Can you work these out from the model? Positions are in its coordinate system, mm. Face numbers are marked on the shaded views. Give positions to 0.01 mm unless a question says otherwise; leave off trailing zeros. Order: outer loops, then holes, each group sorted by start corner. A loop starts at its lowest first (then second) coordinate and runs counter-clockwise, first axis right, second up. Notation, with made-up numbers: (32, -27) - (61, -27) arc R18 ccw to (61, 8) - close; hole circle Ø3 at (-7.75, 84.25). An arc over 180 degrees is marked (long way). Use one line per item in the form item = value. Start each with the question number.
1) We'd pull the mould along X, two halves only. Please class the marked faces 1 and 2: released by +X, released by -X, zero draft, split by the parting line, or undercut.
2) For pin 1 (5 mm diameter, centred on x = 200, z = -85, fed in from +Y); pin 2 (9 mm diameter, centred on x = 404.2, z = -85, fed in from -Y), each with a flat end and sliding along its axis, tell me the tip position at first contact or that it passes through.
3) Suppose I cut it at A-A, the plane z = -65. Write out the boundary of the cut face in (x, y).
4) Suppose I cut it at B-B, the plane x = 52.5. Write out the boundary of the cut face in (y, z), and give its area (3 significant figures).
5) Please list where these lines run through material, in increasing order: probe 1 along X at (y, z) = (5.75, -15); probe 2 along X at (y, z) = (-1.75, -74.5); probe 3 along Z at (x, y) = (200, 6).
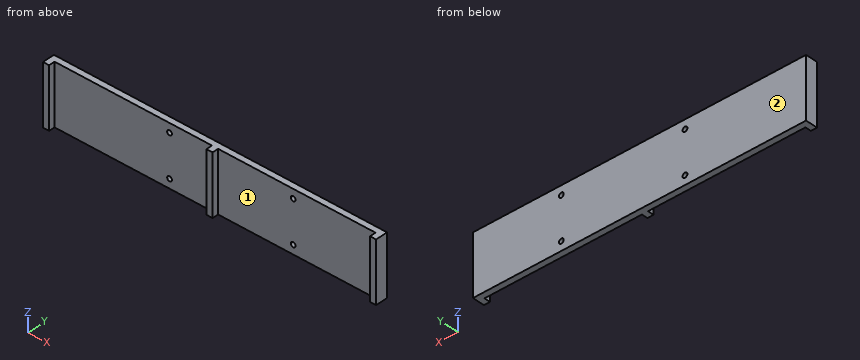
```python
from build123d import *

# Parameters (mm, degrees)
SCHIZZO1_W                   = 550
SCHIZZO1_H                   = 100
SCHIZZO1_R                   = 4
ESTRUSIONE_ESTRUSIONE1_DEPTH = 10
SCHIZZO2_W                   = 10
SCHIZZO2_H                   = 100
ESTRUSIONE_ESTRUSIONE2_DEPTH = 10


with BuildPart() as part:
    # Schizzo1 → Estrusione-Estrusione1 (new body)
    with BuildSketch(Plane(origin=(0, 0, 0), x_dir=(1, 0, 0), z_dir=(0, 1, 0))):
        with Locations((275, 50)):
            Rectangle(SCHIZZO1_W, SCHIZZO1_H)
        with Locations((200, 85)):
            Circle(SCHIZZO1_R, mode=Mode.SUBTRACT)
        with Locations((200, 15)):
            Circle(SCHIZZO1_R, mode=Mode.SUBTRACT)
        with Locations((404.2, 15)):
            Circle(SCHIZZO1_R, mode=Mode.SUBTRACT)
        with Locations((404.2, 85)):
            Circle(SCHIZZO1_R, mode=Mode.SUBTRACT)
    extrude(amount=ESTRUSIONE_ESTRUSIONE1_DEPTH)

    # Schizzo2 → Estrusione-Estrusione2 (add)
    with BuildSketch(Plane.XZ):
        with Locations((5, -50)):
            Rectangle(SCHIZZO2_W, SCHIZZO2_H)
        with Locations((545, -50)):
            Rectangle(SCHIZZO2_W, SCHIZZO2_H)
        with Locations((275, -50)):
            Rectangle(SCHIZZO2_W, SCHIZZO2_H)
    extrude(amount=ESTRUSIONE_ESTRUSIONE2_DEPTH)


solid = part.part
```
Result sheet:
q1.face_1 = undercut
q1.face_2 = zero draft
q2.pin_1 = through
q2.pin_2 = 0
q3.outline = (0, -10) - (10, -10) - (10, 0) - (270, 0) - (270, -10) - (280, -10) - (280, 0) - (540, 0) - (540, -10) - (550, -10) - (550, 10) - (0, 10) - close
q4.outline = (0, -100) - (10, -100) - (10, 0) - (0, 0) - close
q4.area = 1,000 mm²
q5.probe_1 = 0 to 196, 204 to 400.2, 408.2 to 550
q5.probe_2 = 0 to 10, 270 to 280, 540 to 550
q5.probe_3 = -100 to -89, -81 to -19, -11 to 0
